from build123d import *

# Parameters (mm, degrees)
F1_DEPTH = 50
F2_R     = 9.097272


with BuildPart() as f1:
    # F0 (on Right) → F1 (new body)
    with BuildSketch(Plane.YZ):
        with BuildLine():
            ThreePointArc((31.588309, 42.371733), (47.236881, 23.703631), (52.850592, 0))
            ThreePointArc((52.850592, 0), (37.121585, -37.618785), (-0.703132, -52.845914))
            ThreePointArc((-0.703132, -52.845914), (1.366054, -64.640751), (4.641868, -76.158942))
            ThreePointArc((4.641868, -76.158942), (55.569359, -52.285541), (76.300272, 0))
            ThreePointArc((76.300272, 0), (69.417814, 31.668573), (50.012069, 57.623992))
            ThreePointArc((50.012069, 57.623992), (40.405478, 50.474648), (31.588309, 42.371733))
        make_face()
        with BuildLine():
            ThreePointArc((-0.703132, -52.845914), (-50.050711, 16.973845), (31.588309, 42.371733))
            ThreePointArc((31.588309, 42.371733), (40.405478, 50.474648), (50.012069, 57.623992))
            ThreePointArc((50.012069, 57.623992), (-72.25809, 24.505099), (4.641868, -76.158942))
            ThreePointArc((4.641868, -76.158942), (1.366054, -64.640751), (-0.703132, -52.845914))
        make_face()
    extrude(amount=F1_DEPTH)

    # F2
    f2_edges = [f1.edges().sort_by_distance(p)[0] for p in [
        (50, -4.641868, 76.158942),
        (50, -31.588309, -42.371733),
    ]]
    fillet(f2_edges, radius=F2_R)


solid = f1.part
CAD build for the part. Positions are in the model's coordinates, mm. Coordinates: 2 decimals unless noted, no trailing zeros. Write each loop counter-clockwise with the first axis right and the second up, starting at its lowest first coordinate (ties: lowest second). Pieces come first, ordered by that corner, then holes. Notation, with made-up numbers: (-15.5, 35.25) - (31.5, 35.25) arc R22 ccw to (31.5, 47.25) - close; hole circle Ø10 at (-14.75, 47.5). An arc over 180 degrees is marked (long way). Use a Markdown table: item, result. Add a question column.
Item 1: Band-saw the part on A-A, the plane x = 30. Give the cut face in (y, z).
Item 2: Flat gauge pins, fed straight in: pin 1 (8 mm diameter, centred on x = 43.5, z = -29, fed in from +Y); pin 2 (10 mm diameter, centred on x = 36.5, y = -48, fed in from +Z); pin 3 (4 mm diameter, centred on x = 15.5, y = 12, fed in from -Z). Where does each tip first touch, or does it go through?
Item 3: Drill centre lines: L1, parallel to Z at x = 13, y = 0; L2, parallel to Y at x = 6, z = 41.5; L3, parallel to Y at x = 28.5, z = -6. Where is each one in solid material? Low to high. Write a range as from..to.
Numbers:
| question | item | result |
|---|---|---|
| 1 | outline | (50.01, 57.62) arc R76.3 ccw (long way) to (76.3, 0) arc R76.3 ccw to start; hole circle Ø105.7 at (0, 0) |
| 2 | pin 1 | y = 71.92 |
| 2 | pin 2 | z = 63.03 |
| 2 | pin 3 | z = -75.64 |
| 3 | L1 | -76.3..-52.85, 52.85..76.3 |
| 3 | L2 | -64.03..-32.73, 32.73..64.03 |
| 3 | L3 | -76.06..-52.51, 52.51..76.06 |
